Geometry check sheet. Reference: the model listing, model coordinates, mm. A direction names the side the tool comes from. Give positions to 0.01 mm unless a question says otherwise; leave off trailing zeros. Order: outer loops, then holes, each group sorted by start corner. A loop starts at its lowest first (then second) coordinate and runs counter-clockwise, first axis right, second up. Notation, with made-up numbers: M 13.25,-16.5 L 53.25,-16.5 A25 cw 53.25,9.5 Z; hole C 52,2 d7. An arc over 180 degrees is marked long. Answer as CSV lines item,"result". Start each with the question number.
Q1. Section check A-A, the plane x = -68.5. Record the boundary of the cut face in (y, z).
Q2. Section check C-C, the plane x = -107. Record the boundary of the cut face in (y, z).
Q3. Go/stop test with flat-tipped pins: pin 1 (1 mm diameter, centred on y = -0.5, z = -154, fed in from -X); pin 2 (1 mm diameter, centred on x = -64.5, y = 1, fed in from -Z). Record where each tip stops, or that it passes through.
Q4. Thickness scan on line 1 (X direction, y = -0.3, z = -59); line 2 (X direction, y = 1.5, z = -161); line 3 (Z direction, x = -3, y = 0). Record the ranges inside material, lowest first.
Q5. Set-up check for faces 1 (the flat face through (15, 0, -207)), 2 (the flat face through (-49, -2.5, -106)), 3 (the flat face through (14, 0, -3)): record each of +Z, -Z, +X, -X, +Y, -Y from which the full face is reachable in a straight line by a thin tool's end or side.
```python
from build123d import *

# Parameters (mm, degrees)
BOSS_EXTRUDE1_DEPTH      = 2.5
BOSS_EXTRUDE1_DEPTH_BACK = 2.5
SKETCH2_R                = 51.95
CUT_EXTRUDE1_DEPTH       = 245.399774959
SKETCH3_R                = 80.75
CUT_EXTRUDE2_DEPTH       = 3
CUT_EXTRUDE3_START       = -3
SKETCH4_R                = 80.75
CUT_EXTRUDE3_DEPTH       = 3


with BuildPart() as part:
    # Sketch1 → Boss-Extrude1 (new, two sides: drawn at the far end of the back side and taken through both)
    with BuildSketch(Plane(origin=(0, 0, 0), x_dir=(1, 0, 0), z_dir=(0, 1, 0)).offset(-BOSS_EXTRUDE1_DEPTH_BACK)):
        Polygon((-125, 150), (-125, 0), (0, 0), (80.75, 0), (80.75, 210), (0, 210), align=None)
    extrude(amount=BOSS_EXTRUDE1_DEPTH + BOSS_EXTRUDE1_DEPTH_BACK)

    # Sketch2 → Cut-Extrude1 (cut, through all)
    with BuildSketch(Plane(origin=(0, 0, -210), x_dir=(-1, 0, 0), z_dir=(0, 0, -1))):
        with Locations((-80.75, 0)):
            Circle(SKETCH2_R)
    extrude(amount=-CUT_EXTRUDE1_DEPTH, mode=Mode.SUBTRACT)

    # Sketch3 → Cut-Extrude2 (cut)
    with BuildSketch(Plane(origin=(0, 0, -210), x_dir=(-1, 0, 0), z_dir=(0, 0, -1))):
        with Locations((-80.75, 0)):
            Circle(SKETCH3_R)
    extrude(amount=-CUT_EXTRUDE2_DEPTH, mode=Mode.SUBTRACT)

    # Sketch4 → Cut-Extrude3 (cut)
    with BuildSketch(Plane.XY.offset(CUT_EXTRUDE3_START)):
        with Locations((80.75, 0)):
            Circle(SKETCH4_R)
    extrude(amount=CUT_EXTRUDE3_DEPTH, mode=Mode.SUBTRACT)


solid = part.part
```
Answer block:
1,outline,"M -2.5,-177.12 L 2.5,-177.12 L 2.5,0 L -2.5,0 Z"
2,outline,"M -2.5,-158.64 L 2.5,-158.64 L 2.5,0 L -2.5,0 Z"
3,pin 1,"stops at x = -117.71"
3,pin 2,"stops at z = -179.28"
4,line 1,"x = -125 to 28.8"
4,line 2,"x = -102.08 to 28.82"
4,line 3,"z = -208.56 to 0"
5,face 1,"-Z, +X, +Y, -Y"
5,face 2,"+Z, -Z, +X, -X, -Y"
5,face 3,"+Z, +X, +Y, -Y"
